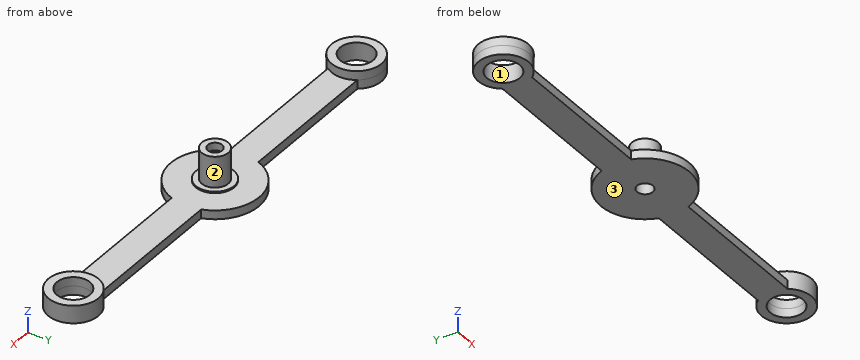
```python
from build123d import *

# Parameters (mm, degrees)
SKETCH1_R               = 4.5
BOSS_EXTRUDE1_DEPTH     = 11
SKETCH2_R               = 5.6
BOSS_EXTRUDE2_DEPTH     = 3
SKETCH3_R               = 6.5
BOSS_EXTRUDE3_DEPTH     = 0.5
SKETCH4_R               = 8.5
SKETCH4_R_2             = 5.6
BOSS_EXTRUDE4_DEPTH     = 3
CUT_EXTRUDE1_START      = 11
SKETCH5_R               = 2.45
CUT_EXTRUDE1_DEPTH      = 2.6
SKETCH7_R               = 1.2
CUT_EXTRUDE3_DEPTH      = 12
CUT_EXTRUDE3_DEPTH_BACK = 4
CUT_EXTRUDE4_START      = -3
SKETCH8_R               = 2.7
CUT_EXTRUDE4_DEPTH      = 8.9


with BuildPart() as part:
    # Sketch1 → Boss-Extrude1 (new body)
    with BuildSketch(Plane.XY):
        Circle(SKETCH1_R)
    extrude(amount=BOSS_EXTRUDE1_DEPTH)

    # Sketch2 → Boss-Extrude2 (add)
    with BuildSketch(Plane.XY):
        with BuildLine():
            Line((14.142135624, 5), (63.126136458, 5))
            ThreePointArc((63.126136458, 5), (78.5, 0), (63.126136458, -5))
            Line((63.126136458, -5), (14.142135624, -5))
            ThreePointArc((14.142135624, -5), (0, -15), (-14.142135624, -5))
            Line((-14.142135624, -5), (-63.126136458, -5))
            ThreePointArc((-63.126136458, -5), (-78.5, 0), (-63.126136458, 5))
            Line((-63.126136458, 5), (-14.142135624, 5))
            ThreePointArc((-14.142135624, 5), (0, 15), (14.142135624, 5))
        make_face()
        with Locations((70, 0)):
            Circle(SKETCH2_R, mode=Mode.SUBTRACT)
        with Locations((-70, 0)):
            Circle(SKETCH2_R, mode=Mode.SUBTRACT)
    extrude(amount=-BOSS_EXTRUDE2_DEPTH)

    # Sketch3 → Boss-Extrude3 (add)
    with BuildSketch(Plane.XY):
        Circle(SKETCH3_R)
    extrude(amount=BOSS_EXTRUDE3_DEPTH)

    # Sketch4 → Boss-Extrude4 (add)
    with BuildSketch(Plane.XY):
        with Locations((-70, 0)):
            Circle(SKETCH4_R)
        with Locations((-70, 0)):
            Circle(SKETCH4_R_2, mode=Mode.SUBTRACT)
        with Locations((70, 0)):
            Circle(SKETCH4_R)
        with Locations((70, 0)):
            Circle(SKETCH4_R_2, mode=Mode.SUBTRACT)
    extrude(amount=BOSS_EXTRUDE4_DEPTH)

    # Sketch5 → Cut-Extrude1 (cut)
    with BuildSketch(Plane.XY.offset(CUT_EXTRUDE1_START)):
        Circle(SKETCH5_R)
    extrude(amount=-CUT_EXTRUDE1_DEPTH, mode=Mode.SUBTRACT)

    # Sketch7 → Cut-Extrude3 (cut, two sides)
    with BuildSketch(Plane.XY) as cut_extrude3_sk:
        Circle(SKETCH7_R)
    extrude(amount=CUT_EXTRUDE3_DEPTH, mode=Mode.SUBTRACT)
    extrude(cut_extrude3_sk.sketch, amount=-CUT_EXTRUDE3_DEPTH_BACK, mode=Mode.SUBTRACT)

    # Sketch8 → Cut-Extrude4 (cut)
    with BuildSketch(Plane.XY.offset(CUT_EXTRUDE4_START)):
        Circle(SKETCH8_R)
    extrude(amount=CUT_EXTRUDE4_DEPTH, mode=Mode.SUBTRACT)


solid = part.part
```
Can you work these out from the model? Positions are in its coordinate system, mm. Face numbers are marked on the shaded views. Coordinates: 2 decimals unless noted, no trailing zeros. Write each loop counter-clockwise with the first axis right and the second up, starting at its lowest first coordinate (ties: lowest second). Pieces come first, ordered by that corner, then holes. Notation, with made-up numbers: (27.25, 8.25) - (65.25, 8.25) arc R18 ccw to (65.25, 25.25) - close; hole circle Ø4 at (62.5, 5). An arc over 180 degrees is marked (long way). Return JSON: item names as keys, results as strings.
Q1. Thinking about a two-plate mould opening in Y: for the marked faces 1, 2 and 3, which applies, +Y half, -Y half, draft (parallel to the pull), parting line (faces both ways), or undercut?
Computed values:
{"face 1": "undercut", "face 2": "parting line", "face 3": "draft"}
Q2. If we section it at A-A (x = 70): Please give me the cut outline in (y, z), then the cut area to 3 significant figures.
Computed values:
{"outline": "(-8.5, -3) - (-5.6, -3) - (-5.6, 3) - (-8.5, 3) - close; (5.6, -3) - (8.5, -3) - (8.5, 3) - (5.6, 3) - close", "area": "34.8 mm2"}
Q3. Please list where these lines run through material, in increasing order: L1, parallel to Y at x = 70, z = -1.45; L2, parallel to Y at x = 0, z = 10.4; L3, parallel to Z at x = -17.5, y = -4.25. Write a range as from..to.
Computed values:
{"L1": "y = -8.5..-5.6, 5.6..8.5", "L2": "y = -4.5..-2.45, 2.45..4.5", "L3": "z = -3..0"}
Q4. I'm going to push flat-ended pins straight in: pin 1 Ø5 at (x, z) = (38.5, 4.5) entering from -Y; pin 2 Ø9 at (x, y) = (-15, 3) entering from +Z; pin 3 Ø12 at (x, y) = (9.5, 5.5) entering from +Z; pin 4 Ø8.5 at (x, y) = (-73.5, 2.5) entering from +Z. Where does each tip first touch, or does it pass through?
Computed values:
{"pin 1": "passes through", "pin 2": "stops at z = 0", "pin 3": "stops at z = 0.5", "pin 4": "stops at z = 3"}
Q5. If we section it at B-B (x = -34): Please give me the cut outline in (y, z), then the cut area to 3 significant figures.
Computed values:
{"outline": "(-5, -3) - (5, -3) - (5, 0) - (-5, 0) - close", "area": "30.0 mm2"}
